Design review of the part built by this model. Coordinates are the model's own, in mm. A direction names the side the tool comes from. Give positions to 0.01 mm unless a question says otherwise; leave off trailing zeros. Loops run counter-clockwise (first coordinate to the right, second up) from the corner with the lowest first, then second, coordinate; pieces in that order, holes last. Notation, with made-up numbers: (53, 56) -> (97, 56) arc R33 cw to (97, 87) -> close; hole circle Ø11 at (-27.5, -35). An arc over 180 degrees is marked (long way). Answer as CSV lines item,"result".
from build123d import *

# Parameters (mm, degrees)
EXTRUDE_1_DEPTH           = 25
CUT_EXTRUDE_4_DEPTH       = 80.457942189
SKETCH_7_W                = 16.60831278
SKETCH_7_H                = 38.473598513
CUT_EXTRUDE_14_DEPTH      = 80.457942189
SKETCH_8_W                = 5
SKETCH_8_H                = 30.968526609
EXTRUDE_2_DEPTH           = 25
CUT_EXTRUDE_15_DEPTH      = 78.792556685
CUT_EXTRUDE_15_DEPTH_BACK = 78.792556685
SKETCH_9_W                = 33.026813651
SKETCH_9_H                = 5
EXTRUDE_3_DEPTH           = 30.968526609
FILLET_1_R                = 3
FILLET_2_R                = 1
SKETCH_11_W               = 2
SKETCH_11_H               = 5
CUT_EXTRUDE_16_DEPTH      = 79.029254622


with BuildPart() as part:
    # Эскиз1 → Бобышка-Вытянуть1 (new body)
    with BuildSketch(Plane(origin=(0, 0, 0), x_dir=(1, 0, 0), z_dir=(0, 1, 0))):
        Polygon((-66.825757576, 34.969739794), (-66.825757576, 29.969739794), (-63.825757576, 29.969739794), (-63.825757576, 31.969739794), (-38.825757576, 31.969739794), (-38.825757576, 6.969739794), (-63.825757576, 6.969739794), (-63.825757576, 8.969739794), (-66.825757576, 8.969739794), (-66.825757576, 3.969739794), (-22.123470102, 3.969739794), (-36.579007505, 34.969739794), align=None)
    extrude(amount=EXTRUDE_1_DEPTH)

    # Эскиз3 → Вырез-Вытянуть4 (cut, through all)
    with BuildSketch(Plane.XZ):
        Polygon((-66.825757576, -3.969739794), (-65.325757576, -8.969739794), (-66.825757576, -8.969739794), align=None)
        Polygon((-66.825757576, -29.969739794), (-66.825757576, -34.969739794), (-65.325757576, -29.969739794), align=None)
    extrude(amount=-CUT_EXTRUDE_4_DEPTH, mode=Mode.SUBTRACT)

    # Эскиз7 → Вырез-Вытянуть14 (cut, through all)
    with BuildSketch(Plane(origin=(0, 0, 0), x_dir=(-1, 0, 0), z_dir=(0, -1, 0))):
        with Locations((27.703474463, 20.539743139)):
            Rectangle(SKETCH_7_W, SKETCH_7_H)
    extrude(amount=-CUT_EXTRUDE_14_DEPTH, mode=Mode.SUBTRACT)

    # Эскиз8 → Бобышка-Вытянуть2 (add)
    with BuildSketch(Plane(origin=(0, 0, 0), x_dir=(-1, 0, 0), z_dir=(0, -1, 0))):
        with Locations((36.298943925, 19.454003098)):
            Rectangle(SKETCH_8_W, SKETCH_8_H)
    extrude(amount=-EXTRUDE_2_DEPTH)

    # Эскиз9 → Вырез-Вытянуть15 (cut, two sides: drawn at the far end of the back side and taken through both)
    with BuildSketch(Plane.XY.offset(-3.969739794).offset(-CUT_EXTRUDE_15_DEPTH_BACK)):
        with Locations((-50.312350751, 2.5)):
            Rectangle(SKETCH_9_W, SKETCH_9_H)
    extrude(amount=CUT_EXTRUDE_15_DEPTH + CUT_EXTRUDE_15_DEPTH_BACK, mode=Mode.SUBTRACT)

    # Эскиз10 → Бобышка-Вытянуть3 (add)
    with BuildSketch(Plane.XY.offset(-3.969739794)):
        with BuildLine():
            Line((-26.798943925, 18.714044563), (-25.41833427, 20.714562355))
            ThreePointArc((-25.41833427, 20.714562355), (-36.206138223, 14.922403986), (-25.290934081, 9.374059074))
            Line((-25.290934081, 9.374059074), (-26.798943925, 11.285955437))
            ThreePointArc((-26.798943925, 11.285955437), (-33.776010712, 15), (-26.798943925, 18.714044563))
        make_face()
    extrude(amount=-EXTRUDE_3_DEPTH)

    # Скругление1
    fillet_1_edges = [part.edges().sort_by_distance(p)[0] for p in [
        (-33.798943925, 9.759260146, -19.454003099),
        (-33.798943925, 20.240739854, -19.454003099),
    ]]
    fillet(fillet_1_edges, radius=FILLET_1_R)

    # Скругление2
    fillet_2_edges = [part.edges().sort_by_distance(p)[0] for p in [
        (-25.41833427, 20.714562355, -19.454003099),
        (-25.290934081, 9.374059074, -19.454003099),
    ]]
    fillet(fillet_2_edges, radius=FILLET_2_R)

    # Эскиз11 → Вырез-Вытянуть16 (cut, through all)
    with BuildSketch(Plane.XZ.offset(-5)):
        with Locations((-32.798943925, -12.244728029)):
            Rectangle(SKETCH_11_W, SKETCH_11_H)
        with Locations((-32.798943925, -29.654311708)):
            Rectangle(SKETCH_11_W, SKETCH_11_H)
    extrude(amount=-CUT_EXTRUDE_16_DEPTH, mode=Mode.SUBTRACT)


solid = part.part
Q1. Clearance check with flat-ended pins moving along their axes: pin 1 Ø3.5 at (y, z) = (9, -13) entering from -X; pin 2 Ø8 at (x, z) = (-46, -25) entering from -Y; pin 3 Ø0.6 at (y, z) = (12, -8.5) entering from +X; pin 4 Ø2 at (x, y) = (-33.5, 18.5) entering from -Z. State where each tip first meets the part, or that it passes through.
Filled sheet:
pin 1,"stops at x = -38.83"
pin 2,"passes through"
pin 3,"stops at x = -32.32"
pin 4,"stops at z = -34.94"
Q2. For faces 4 (the flat face through (-66.086, 14.86, -32.505)), 5 (the cylindrical face through (-25.903, 20.661, -19.671)), 6 (the flat face through (-31.799, 20, -12)), list the 3-axis set-ups (+Z, -Z, +X, -X, +Y, -Y) from which the entire face can be reached by the end or side of a thin tool; tool diameter is ignored.
Filled sheet:
face 4,"-X, +Y, -Y"
face 5,"+Z, -Z, +X"
face 6,"+Y, -Y"
Q3. We need section D-D, the plane z = -18. State the section outline as (x, y) points.
Filled sheet:
outline,"(-38.83, 5) -> (-33.8, 5) -> (-33.8, 5.21) arc R3 cw to (-30.34, 8.17) arc R6.91 ccw to (-26.36, 8.75) arc R1 ccw to (-26, 10.27) -> (-26.8, 11.29) arc R4.48 cw (long way) to (-26.8, 18.71) -> (-26.04, 19.81) arc R1 ccw to (-26.45, 21.29) arc R6.91 ccw to (-30.34, 21.83) arc R3 cw to (-33.8, 24.79) -> (-33.8, 25) -> (-38.83, 25) -> close"
Q4. The part is to be moulded in two halves that separate along X. For faces 1 (the flat face through (-26.42, 19.26, -19.24)), 2 (the flat face through (-33.5, 12.7, -9.745)), 3 (the flat face through (-51, 15, -3.97)), say which applies: pulls with the +X half, pulls with the -X half, needs draft (parallel to the pull), parting line crosses it, or undercut.
Filled sheet:
face 1,"pulls with the +X half"
face 2,"undercut"
face 3,"needs draft"
Q5. We need section B-B, the plane z = -14. State the section outline as (x, y) points (3 decimals).
Filled sheet:
outline,"(-38.826, 5) -> (-33.799, 5) -> (-33.799, 25) -> (-38.826, 25) -> close; (-31.799, 8.035) arc R3 cw to (-30.345, 8.172) arc R6.908 ccw to (-26.36, 8.749) arc R1 ccw to (-26, 10.273) -> (-26.799, 11.286) arc R4.477 cw to (-31.799, 11.286) -> close; (-31.799, 18.714) arc R4.477 cw to (-26.799, 18.714) -> (-26.04, 19.814) arc R1 ccw to (-26.451, 21.293) arc R6.908 ccw to (-30.345, 21.828) arc R3 cw to (-31.799, 21.965) -> close"
Q6. We need section A-A, the plane x = -46. State the section outline as (y, z) points, and give its area (3 significant figures).
Filled sheet:
outline,"(5, -34.97) -> (25, -34.97) -> (25, -31.97) -> (5, -31.97) -> close; (5, -6.97) -> (25, -6.97) -> (25, -3.97) -> (5, -3.97) -> close"
area,"120 mm^2"
Q7. To check wall thickness, follow probe 1 along Z at (x, y) = (-33.5, 19); probe 2 along Z at (x, y) = (-47.5, 8); probe 3 along Z at (x, y) = (-64, 12). State the ranges of each line that lie inside material, in increasing order. Write a range as from..to.
Filled sheet:
probe 1,"z = -34.94..-32.15, -27.15..-14.74, -9.74..-3.97"
probe 2,"z = -34.97..-31.97, -6.97..-3.97"
probe 3,"z = -34.97..-29.97, -8.97..-3.97"
